```python
from build123d import *

# Parameters (mm, degrees)
SKETCH1_W           = 133
SKETCH1_H           = 102
SKETCH1_R           = 14.225
SKETCH1_R_2         = 1.25
SKETCH1_R_3         = 8
BOSS_EXTRUDE2_DEPTH = 4.7625
CUT_EXTRUDE1_REACH  = 113.1
SKETCH2_R           = 3.18


with BuildPart() as part:
    # Sketch1 → Boss-Extrude2 (new body)
    with BuildSketch(Plane.XY):
        with Locations((-18.535460993, 20.341271178)):
            Rectangle(SKETCH1_W, SKETCH1_H)
        with Locations(Location((-30.035460993, 13.261258957, 0), (0, 0, 180))):
            Circle(SKETCH1_R, mode=Mode.SUBTRACT)
        with Locations(Location((23.965174075, -9.826590747, 0), (0, 0, 180))):
            Circle(SKETCH1_R_2, mode=Mode.SUBTRACT)
        with Locations(Location((37.965174075, 4.173409253, 0), (0, 0, 180))):
            Circle(SKETCH1_R_2, mode=Mode.SUBTRACT)
        with Locations(Location((23.965174075, 18.173409253, 0), (0, 0, 180))):
            Circle(SKETCH1_R_2, mode=Mode.SUBTRACT)
        with Locations(Location((9.965174075, 4.173409253, 0), (0, 0, 180))):
            Circle(SKETCH1_R_2, mode=Mode.SUBTRACT)
        with Locations(Location((23.965174075, 4.173409253, 0), (0, 0, 180))):
            Circle(SKETCH1_R_3, mode=Mode.SUBTRACT)
    extrude(amount=BOSS_EXTRUDE2_DEPTH)

    # Sketch2 → Cut-Extrude1 (cut, up to next)
    with BuildSketch(Plane.XY.offset(4.7625), mode=Mode.PRIVATE) as cut_extrude1_sk1:
        with Locations((-70.035460993, 61.341271178)):
            Circle(SKETCH2_R)
    cut_extrude1_tool1 = extrude(cut_extrude1_sk1.sketch, amount=-CUT_EXTRUDE1_REACH, mode=Mode.PRIVATE) & part.part
    # Sketch2 → Cut-Extrude1 (cut, up to next)
    with BuildSketch(Plane.XY.offset(4.7625), mode=Mode.PRIVATE) as cut_extrude1_sk2:
        with Locations((32.964539007, 46.341271178)):
            Circle(SKETCH2_R)
    cut_extrude1_tool2 = extrude(cut_extrude1_sk2.sketch, amount=-CUT_EXTRUDE1_REACH, mode=Mode.PRIVATE) & part.part
    # Sketch2 → Cut-Extrude1 (cut, up to next)
    with BuildSketch(Plane.XY.offset(4.7625), mode=Mode.PRIVATE) as cut_extrude1_sk3:
        with Locations((11.964539007, -23.658728822)):
            Circle(SKETCH2_R)
    cut_extrude1_tool3 = extrude(cut_extrude1_sk3.sketch, amount=-CUT_EXTRUDE1_REACH, mode=Mode.PRIVATE) & part.part
    # Sketch2 → Cut-Extrude1 (cut, up to next)
    with BuildSketch(Plane.XY.offset(4.7625), mode=Mode.PRIVATE) as cut_extrude1_sk4:
        with Locations((-78.035460993, -23.658728822)):
            Circle(SKETCH2_R)
    cut_extrude1_tool4 = extrude(cut_extrude1_sk4.sketch, amount=-CUT_EXTRUDE1_REACH, mode=Mode.PRIVATE) & part.part
    add(cut_extrude1_tool1.solids().sort_by_distance((-70.035461, 61.341271, 4.7625))[0], mode=Mode.SUBTRACT)
    add(cut_extrude1_tool2.solids().sort_by_distance((32.964539, 46.341271, 4.7625))[0], mode=Mode.SUBTRACT)
    add(cut_extrude1_tool3.solids().sort_by_distance((11.964539, -23.658729, 4.7625))[0], mode=Mode.SUBTRACT)
    add(cut_extrude1_tool4.solids().sort_by_distance((-78.035461, -23.658729, 4.7625))[0], mode=Mode.SUBTRACT)


solid = part.part
```
Verification items for the finished model (mm, model axes). Give positions to 0.01 mm unless a question says otherwise; leave off trailing zeros. Loops run counter-clockwise (first coordinate to the right, second up) from the corner with the lowest first, then second, coordinate; pieces in that order, holes last. Notation, with made-up numbers: M 41,1 L 64,1 A28 ccw 64,21 Z; hole C 44,22 d1. An arc over 180 degrees is marked long. Return JSON: item names as keys, results as strings.
1) Material ranges on L1, parallel to X at y = -26, z = 2.3; L2, parallel to X at y = 18.5, z = 2.95; L3, parallel to Y at x = 11.5, z = 3.95, recorded low to high. Write a range as [from, to].
Findings:
{"L1": "x = [-85.04, -80.19], [-75.88, 9.81], [14.12, 47.96]", "L2": "x = [-85.04, -43.26], [-16.81, 22.76], [25.17, 47.96]", "L3": "y = [-30.66, -26.8], [-20.51, 71.34]"}
2) Section check B-B, the plane x = -30.5. Enter the section's corners in (y, z).
Findings:
{"outline": "M -30.66,0 L -0.96,0 L -0.96,4.76 L -30.66,4.76 Z; M 27.48,0 L 71.34,0 L 71.34,4.76 L 27.48,4.76 Z"}
3) Mould release check, pull along X, two halves, no side actions. Record for faces 1 (the cylindrical face through (-67.1, 60.12, 2.41)), 2 (the flat face through (-85.035, 20, 2)), 3 (the flat face through (47.965, 20, 2)): released by +X, released by -X, zero draft, split by the parting line, or undercut.
Findings:
{"face 1": "undercut", "face 2": "released by -X", "face 3": "released by +X"}
4) Section check A-A, the plane y = 0.5. Enter the section's corners in (x, z).
Findings:
{"outline": "M -85.04,0 L -36.32,0 L -36.32,4.76 L -85.04,4.76 Z; M -23.75,0 L 16.86,0 L 16.86,4.76 L -23.75,4.76 Z; M 31.07,0 L 47.96,0 L 47.96,4.76 L 31.07,4.76 Z"}
5) Section check C-C, the plane y = 15. Enter the section's corners in (x, z).
Findings:
{"outline": "M -85.04,0 L -44.15,0 L -44.15,4.76 L -85.04,4.76 Z; M -15.92,0 L 47.96,0 L 47.96,4.76 L -15.92,4.76 Z"}
6) Section check D-D, the plane z = 3.65. Count the separate pieces of the cut face and the enclosed holes in it, and give its area (3 significant figures).
Findings:
{"separate pieces": "1", "enclosed holes": "10", "area": "12,600 mm2"}
